```python
from build123d import *

# Parameters (mm, degrees)
SKETCH_1_R          = 1.6
SKETCH_1_R_2        = 2
SKETCH_1_R_3        = 13.1
EXTRUDE_1_DEPTH     = 3
SKETCH_2_R          = 2.1
CUT_EXTRUDE_1_DEPTH = 117.253215009
FILLET_1_R          = 10
SKETCH_4_W          = 19.6
SKETCH_4_H          = 26.07233047
SKETCH_4_W_2        = 46
SKETCH_4_H_2        = 14.67766953
CUT_EXTRUDE_2_DEPTH = 117.253215009
FILLET_2_R          = 3


with BuildPart() as part:
    # 草图1 → 凸台-拉伸1 (new body)
    with BuildSketch(Plane.XY):
        Polygon((0, 0), (0, 77.5), (60, 77.5), (60, 57.5), (86.6, 57.5), (86.6, 0), align=None)
        with Locations((12.32233047, 42.5)):
            Circle(SKETCH_1_R, mode=Mode.SUBTRACT)
        with Locations((30, 42.32233047)):
            Circle(SKETCH_1_R_2, mode=Mode.SUBTRACT)
        with Locations((30, 24.82233047)):
            Circle(SKETCH_1_R_3, mode=Mode.SUBTRACT)
        with Locations((12.5, 24.82233047)):
            Circle(SKETCH_1_R_2, mode=Mode.SUBTRACT)
        with Locations((12.32233047, 7.144660941)):
            Circle(SKETCH_1_R, mode=Mode.SUBTRACT)
        with Locations((30, 7.32233047)):
            Circle(SKETCH_1_R_2, mode=Mode.SUBTRACT)
        with Locations((47.67766953, 7.144660941)):
            Circle(SKETCH_1_R, mode=Mode.SUBTRACT)
        with Locations((47.5, 24.82233047)):
            Circle(SKETCH_1_R_2, mode=Mode.SUBTRACT)
        with Locations((47.67766953, 42.5)):
            Circle(SKETCH_1_R, mode=Mode.SUBTRACT)
    extrude(amount=EXTRUDE_1_DEPTH)

    # 草图2 → 切除-拉伸1 (cut, through all)
    with BuildSketch(Plane.XY.offset(3)):
        with Locations((10, 67.5)):
            Circle(SKETCH_2_R)
        with Locations((50, 67.5)):
            Circle(SKETCH_2_R)
        with Locations((76.6, 48.75)):
            Circle(SKETCH_2_R)
        with Locations((76.6, 8.75)):
            Circle(SKETCH_2_R)
    extrude(amount=-CUT_EXTRUDE_1_DEPTH, mode=Mode.SUBTRACT)

    # 圆角1
    fillet_1_edges = [part.edges().sort_by_distance(p)[0] for p in [
        (0, 77.5, 1.5),
        (0, 0, 1.5),
        (86.6, 0, 1.5),
        (86.6, 57.5, 1.5),
        (60, 77.5, 1.5),
        (60, 57.5, 1.5),
    ]]
    fillet(fillet_1_edges, radius=FILLET_1_R - 0.0001)  # a hair under: the kernel refuses the full size

    # 草图4 → 切除-拉伸2 (cut, through all)
    with BuildSketch(Plane.XY.offset(3)):
        with Locations((61.8, 27.786165235)):
            Rectangle(SKETCH_4_W, SKETCH_4_H)
        with Locations((33, 54.161165235)):
            Rectangle(SKETCH_4_W_2, SKETCH_4_H_2)
    extrude(amount=-CUT_EXTRUDE_2_DEPTH, mode=Mode.SUBTRACT)

    # 圆角2
    fillet_2_edges = [part.edges().sort_by_distance(p)[0] for p in [
        (56, 46.82233047, 1.5),
        (10, 46.82233047, 1.5),
        (10, 61.5, 1.5),
        (56, 61.5, 1.5),
        (52, 14.75, 1.5),
        (52, 40.82233047, 1.5),
        (71.6, 40.82233047, 1.5),
        (71.6, 14.75, 1.5),
    ]]
    fillet(fillet_2_edges, radius=FILLET_2_R)


solid = part.part
```
CAD build for the part. Positions are in the model's coordinates, mm. A direction names the side the tool comes from. Coordinates: 2 decimals unless noted, no trailing zeros. Write each loop counter-clockwise with the first axis right and the second up, starting at its lowest first coordinate (ties: lowest second). Pieces come first, ordered by that corner, then holes.
(1) Flat gauge pins, fed straight in: pin 1 (1.5 mm diameter, centred on x = 58.5, z = 2, fed in from +Y); pin 2 (5.5 mm diameter, centred on x = 10, y = 67.5, fed in from +Z). Where does each tip first touch, or does it go through?
(2) Cut at D-D, the plane y = 72. List the corners of the cut face in (x, z), and give its area (3 significant figures).
(3) Cut at A-A, the plane y = 30. List the corners of the cut face in (x, z), and give its area (3 significant figures).
(4) Drill centre lines: probe 1 along Y at (x, z) = (30, 2.55); probe 2 along Y at (x, z) = (16.5, 0.25); probe 3 along X at (y, z) = (23, 0.35). Where is each one in solid material? Low to high.
(5) Cut at B-B, the plane x = 54. List the corners of the cut face in (y, z), and give its area (3 significant figures).
(6) 3-axis set-ups, long thin cutter, end or side, ignore diameter. For faces 4 (the face through (52, 28, 2)), 5 (the face through (44, 39, 0)): which of +Z, -Z, +X, -X, +Y, -Y reach the whole face in a straight line?
(7) Cut at C-C, the plane z = 2.05. Count the separate pieces of the cut face and the enclosed holes in it, and give its area (3 significant figures).
(8) Two-plate mould, pull along X, no slides. Class faces 1 (the face through (44, 0, 1)), 2 (the face through (2.85, 74.49, 1.52)), 3 (the face through (10.9, 60.64, 1.48)): +X half, -X half, draft (parallel to the pull), parting line (faces both ways), or undercut.
Geometry says:
1. pin 1: stops at y = 73.82
1. pin 2: stops at z = 3
2. outline: (1.07, 0) - (58.93, 0) - (58.93, 3) - (1.07, 3) - close
2. area: 174 mm2
3. outline: (0, 0) - (17.97, 0) - (17.97, 3) - (0, 3) - close; (42.03, 0) - (52, 0) - (52, 3) - (42.03, 3) - close; (71.6, 0) - (86.6, 0) - (86.6, 3) - (71.6, 3) - close
3. area: 129 mm2
4. probe 1: y = 0 to 5.32, 9.32 to 11.72, 37.92 to 40.32, 44.32 to 46.82, 61.5 to 77.5
4. probe 2: y = 0 to 46.82, 61.5 to 77.5
4. probe 3: x = 0 to 11.68, 13.32 to 17.03, 42.97 to 46.68, 48.32 to 52, 71.6 to 86.6
5. outline: (0, 0) - (14.92, 0) - (14.92, 3) - (0, 3) - close; (40.65, 0) - (46.99, 0) - (46.99, 3) - (40.65, 3) - close; (61.33, 0) - (76.67, 0) - (76.67, 3) - (61.33, 3) - close
5. area: 110 mm2
6. face 4: +Z, -Z
6. face 5: -Z, +X, -X, +Y, -Y
7. separate pieces: 1
7. enclosed holes: 15
7. area: 4,250 mm2
8. face 1: draft
8. face 2: -X half
8. face 3: undercut
